Answer from the drawing. Dimensions are ordinates in mm from the lowest x, y and z of the part. A direction names the side the tool comes from. Round coordinates to 2 decimals unless told otherwise and drop trailing zeros. Order: outer loops, then holes, each group sorted by start corner. A loop starts at its lowest first (then second) coordinate and runs counter-clockwise, first axis right, second up. Notation, with made-up numbers: (12, 29) - (60, 29) arc R21 cw to (60, 67) - close; hole circle Ø6 at (70, 32.25). An arc over 180 degrees is marked (long way). One line per question, with ' | ' between items. Start each with the question number.
1) The part is cut by section B-B, the plane z = 22. Give the vertices of the cut face in (x, y), plus the area to 3 significant figures.
2) The part is cut by section D-D, the plane x = 75. Give the vertices of the cut face in (y, z).
3) The mould has two halves that part along Z. Classify the marked faces 3, 4, 5 and 6: pulls with the +Z half, pulls with the -Z half, needs draft (parallel to the pull), parting line crosses it, or undercut.
4) Straight lines are drawn through the part: line 1 (X direction, y = 17, z = 16.5); line 2 (Y direction, x = 104, z = 29); line 3 (X direction, y = 21.5, z = 12). For each, find the intervals that lie inside material, in ascending order. Write a range as from..to.
5) For the marked faces 1 and 2, determine the directions among +Z, -Z, +X, -X, +Y, -Y from which every point of the face is accessible in a straight line to the end or side of a thin tool.
6) The part is cut by section C-C, the plane y = 9.5. Give the vertices of the cut face in (x, z) (3 decimals).
7) The part is cut by section A-A, the plane y = 34.5. Give the vertices of the cut face in (x, z) (3 decimals).
8) Flat-ended cylindrical pins translate along their axes: pin 1 (6 mm diameter, centred on x = 60.5, z = 21.5, fed in from -Y); pin 2 (4 mm diameter, centred on y = 6.5, z = 9, fed in from +X); pin 3 (10 mm diameter, centred on y = 9.5, z = 28.5, fed in from +X). Find the tip coordinate at first contact, or state that the pin passes through.
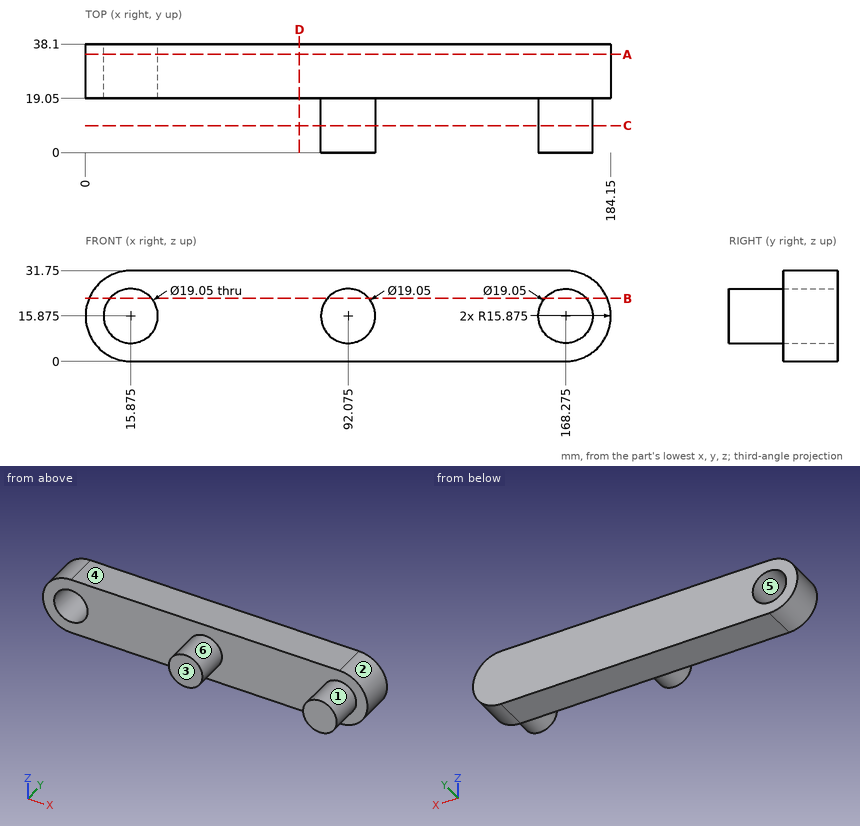
Values:
1) outline: (1.23, 19.05) - (8.58, 19.05) - (8.58, 38.1) - (1.23, 38.1) - close; (23.17, 19.05) - (84.78, 19.05) - (84.78, 0) - (99.37, 0) - (99.37, 19.05) - (160.98, 19.05) - (160.98, 0) - (175.57, 0) - (175.57, 19.05) - (182.92, 19.05) - (182.92, 38.1) - (23.17, 38.1) - close | area: 3,740 mm^2
2) outline: (19.05, 0) - (38.1, 0) - (38.1, 31.75) - (19.05, 31.75) - close
3) face 3: needs draft | face 4: pulls with the +Z half | face 5: undercut | face 6: parting line crosses it
4) line 1: x = 82.57..101.58, 158.77..177.78 | line 2: y = 19.05..38.1 | line 3: x = 0.48..7.17, 24.58..183.67
5) face 1: -Y | face 2: +X, +Y, -Y
6) outline: circle Ø19.05 at (92.075, 15.875); circle Ø19.05 at (168.275, 15.875)
7) outline: (15.875, 0) - (168.275, 0) arc R15.875 ccw to (168.275, 31.75) - (15.875, 31.75) arc R15.875 ccw to start; hole circle Ø19.05 at (15.875, 15.875)
8) pin 1: stops at y = 19.05 | pin 2: stops at x = 176.46 | pin 3: stops at x = 173.98
